The listing builds one solid part. Answer for the finished solid, in the listing's coordinates (mm). A direction names the side the tool comes from. Give positions to 0.01 mm unless a question says otherwise; leave off trailing zeros. Answer as a JSON object with one key per item and string values. Group by question number.
Q1. Given pin 1 (5 mm diameter, centred on x = -17.5, y = 2, fed in from +Z), flat-ended and moving along its own axis, determine where the tip first touches the part or whether it passes through.
Q2. The mould has two halves that part along X. Classify faces 4 (the face through (-40.57, -0.17, -6.56)), 5 (the face through (-44.42, 14.715, 0.059)), 6 (the face through (-10, -15, 0)): released by +X, released by -X, zero draft, split by the parting line, or undercut.
Q3. Consider line 1 (X direction, y = -7.25, z = 13); line 2 (Y direction, x = -21, z = 0); line 3 (X direction, y = -2.5, z = 10). Determine where each line is inside the solid, lowest interval first.
Q4. For faces 1 (the face through (-36.25, -0.17, -3.32)), 2 (the face through (-18, -11.5, 5)), 3 (the face through (25, 0, -1)), determine the directions among +Z, -Z, +X, -X, +Y, -Y from which every point of the face is accessible in a straight line to the end or side of a thin tool.
from build123d import *

# Parameters (mm, degrees)
F1_DEPTH = 15
F3_W     = 8.2
F3_H     = 23
F3_W_2   = 9.5
F3_H_2   = 20.3
F3_W_3   = 9.6
F3_H_3   = 17.9
F3_W_4   = 8.9
F3_H_4   = 19.1
F4_DEPTH = 25
F5_W     = 2.5
F5_H     = 24.5
F6_DEPTH = 15
F7_DEPTH = 15
F8_R     = 1


# Not quite as in the source:
# - a feature names something its author has since deleted; it is built from what else it names


with BuildPart() as f1:
    # F0 (on Front) → F1 (new body, symmetric)
    with BuildSketch(Plane.XZ):
        Polygon((25, -15), (25, 15), (-25, 15), (-65, -15), (-25, -15), align=None)
    extrude(amount=F1_DEPTH, both=True)

    # F3 (on offset) → F4 (cut)
    with BuildSketch(Plane.XY.offset(20)):
        with Locations((-17.9062577261, 0)):
            Rectangle(F3_W, F3_H)
        with Locations((-6.4574469417, 0)):
            Rectangle(F3_W_2, F3_H_2)
        with Locations((5.7595338684, 0)):
            Rectangle(F3_W_3, F3_H_3)
        with Locations((17.6052688631, 0)):
            Rectangle(F3_W_4, F3_H_4)
    extrude(amount=-F4_DEPTH, mode=Mode.SUBTRACT)

    # F5 (on face) → F6 (cut)
    with BuildSketch(Plane(origin=(-16.2, 0, 21.6), x_dir=(0.8, 0, 0.6), z_dir=(-0.6, 0, 0.8))):
        with Locations((-20.6918526966, 0)):
            Rectangle(F5_W, F5_H)
    extrude(amount=-F6_DEPTH, mode=Mode.SUBTRACT)

    # F5 (on face) → F7 (cut)
    with BuildSketch(Plane(origin=(-16.2, 0, 21.6), x_dir=(0.8, 0, 0.6), z_dir=(-0.6, 0, 0.8))):
        with Locations((-26.6418426484, -3.204e-07)):
            Rectangle(F5_W, F5_H)
        with Locations((-32.2418349981, 3.204e-07)):
            Rectangle(F5_W, F5_H)
        with Locations((-37.6418220997, 0)):
            Rectangle(F5_W, F5_H)
    extrude(amount=-F7_DEPTH, mode=Mode.SUBTRACT)

    # F8
    f8_edges = [f1.edges().sort_by_distance(p)[0] for p in [
        (-25, 0, 15),
        (-45, 15, 0),
        (-45, -15, 0),
        (-65, 0, -15),
        (-33.753482, 0, 8.434888),
        (-32.753482, 12.25, 9.184888),
        (-32.753482, -12.25, 9.184888),
        (-31.753482, 0, 9.934888),
        (-41.993468, -12.25, 2.254899),
        (-40.993468, 0, 3.004899),
        (-41.993468, 12.25, 2.254899),
        (-42.993468, 0, 1.504899),
        (-45.313458, 0, -0.235093),
        (-46.313458, 12.25, -0.985093),
        (-47.313458, 0, -1.735093),
        (-46.313458, -12.25, -0.985093),
        (-36.513474, 0, 6.364894),
        (-37.513474, 12.25, 5.614894),
        (-38.513474, 0, 4.864894),
        (-37.513474, -12.25, 5.614894),
        (25, 0, 15),
        (0, 15, 15),
        (0, -15, 15),
        (22.055269, 0, 15),
        (17.605269, 9.55, 15),
        (13.155269, 0, 15),
        (17.605269, -9.55, 15),
        (10.559534, 0, 15),
        (5.759534, 8.95, 15),
        (0.959534, 0, 15),
        (5.759534, -8.95, 15),
        (-11.207447, 0, 15),
        (-6.457447, -10.15, 15),
        (-1.707447, 0, 15),
        (-6.457447, 10.15, 15),
        (-17.906258, -11.5, 15),
        (-13.806258, 0, 15),
        (-17.906258, 11.5, 15),
        (-22.006258, 0, 15),
        (25, -15, 0),
        (25, 15, 0),
    ]]
    fillet(f8_edges, radius=F8_R)


solid = f1.part
Reply:
{
 "1": {"pin 1": "stops at z = -5"},
 "2": {"face 4": "undercut", "face 5": "released by -X", "face 6": "zero draft"},
 "3": {"line 1": "x = -27.67 to -22.01, -13.81 to -11.21, -1.71 to 0.96, 10.56 to 13.16, 22.06 to 25", "line 2": "y = -15 to -11.5, 11.5 to 15", "line 3": "x = -31.32 to -22.01, -13.81 to -11.21, -1.71 to 0.96, 10.56 to 13.16, 22.06 to 25"},
 "4": {"face 1": "none", "face 2": "+Z", "face 3": "+Z, -Z, +X, +Y, -Y"}
}
